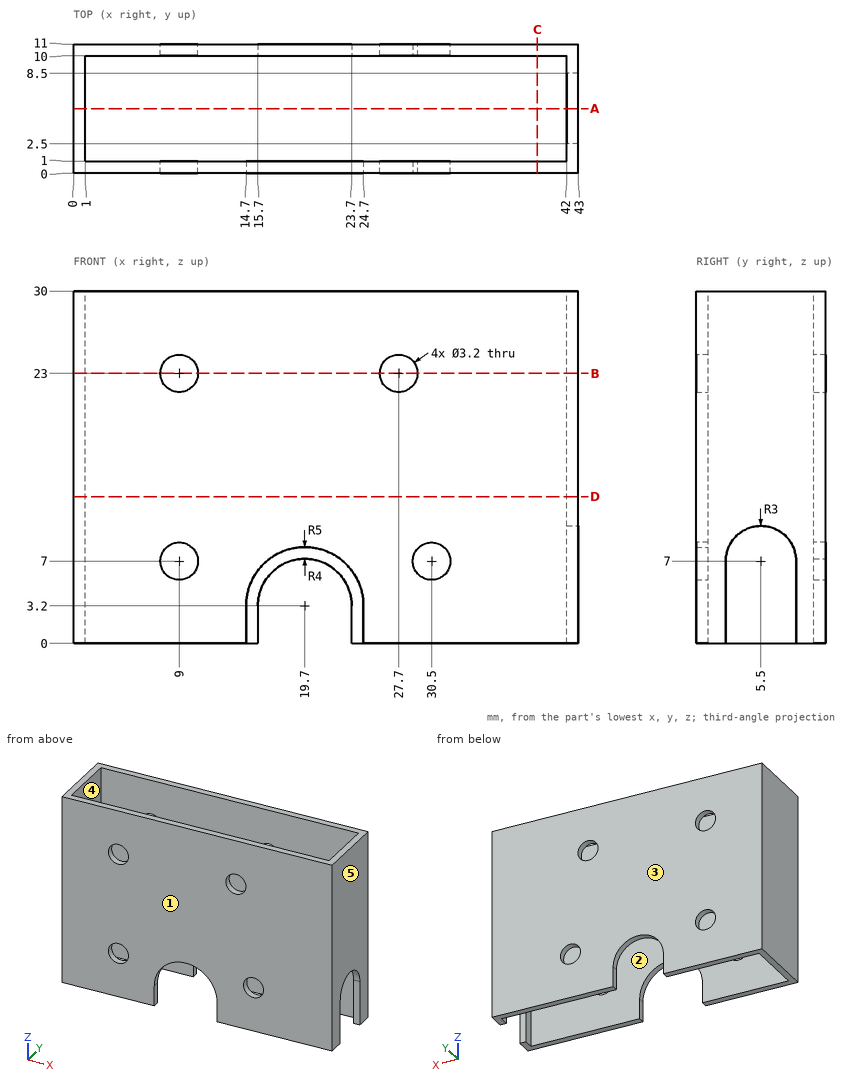
Study the drawing (mm; zero at the part's minimum x, y, z) and answer. A direction names the side the tool comes from. Coordinates: 2 decimals unless noted, no trailing zeros. Write each loop counter-clockwise with the first axis right and the second up, starting at its lowest first coordinate (ties: lowest second). Pieces come first, ordered by that corner, then holes. Notation, with made-up numbers: (75.5, 49) - (124.5, 49) arc R21 cw to (124.5, 83) - close; hole circle Ø6 at (16, 35). An arc over 180 degrees is marked (long way). Answer as a JSON object with one key per item and string values. Group by question number.
1. Consider L1, parallel to X at y = 10.65, z = 23; L2, parallel to Y at x = 33.5, z = 27.5; L3, parallel to X at y = 7.25, z = 24.25. Determine where each line is inside the solid, lowest interval first. Write a range as [from, to].
2. Which of the six approach directions +Z, -Z, +X, -X, +Y, -Y give full straight-line access (tool end or side, diameter ignored) to the marked faces 1 and 2?
3. A cutting plane is placed at A-A (y = 5.5). Determine the outline of the cut face in (x, z), plus the area to 3 significant figures.
4. A cutting plane is placed at C-C (x = 39.5). Determine the outline of the cut face in (y, z).
5. A cutting plane is placed at D-D (z = 12.5). Determine the outline of the cut face in (x, y), plus the area to 3 significant figures.
6. The mould has two halves that part along Y. Classify the marked faces 3, 4 and 5: +Y half, -Y half, draft (parallel to the pull), parting line (faces both ways), or undercut.
7. A cutting plane is placed at B-B (z = 23). Determine the outline of the cut face in (x, y), plus the area to 3 significant figures.
Worked out:
{
 "1": {"L1": "x = [0, 7.4], [10.6, 26.1], [29.3, 43]", "L2": "y = [0, 1], [10, 11]", "L3": "x = [0, 1], [42, 43]"},
 "2": {"face 1": "+Z, -Z, +X, -X, -Y", "face 2": "+Z, -Z"},
 "3": {"outline": "(0, 0) - (1, 0) - (1, 30) - (0, 30) - close; (42, 10) - (43, 10) - (43, 30) - (42, 30) - close", "area": "50.0 mm²"},
 "4": {"outline": "(0, 0) - (1, 0) - (1, 30) - (0, 30) - close; (10, 0) - (11, 0) - (11, 30) - (10, 30) - close"},
 "5": {"outline": "(0, 0) - (43, 0) - (43, 11) - (0, 11) - close; hole (1, 1) - (42, 1) - (42, 10) - (1, 10) - close", "area": "104 mm²"},
 "6": {"face 3": "+Y half", "face 4": "undercut", "face 5": "draft"},
 "7": {"outline": "(0, 0) - (7.4, 0) - (7.4, 1) - (1, 1) - (1, 10) - (7.4, 10) - (7.4, 11) - (0, 11) - close; (10.6, 0) - (26.1, 0) - (26.1, 1) - (10.6, 1) - close; (10.6, 10) - (26.1, 10) - (26.1, 11) - (10.6, 11) - close; (29.3, 0) - (43, 0) - (43, 11) - (29.3, 11) - (29.3, 10) - (42, 10) - (42, 1) - (29.3, 1) - close", "area": "91.2 mm²"}
}
